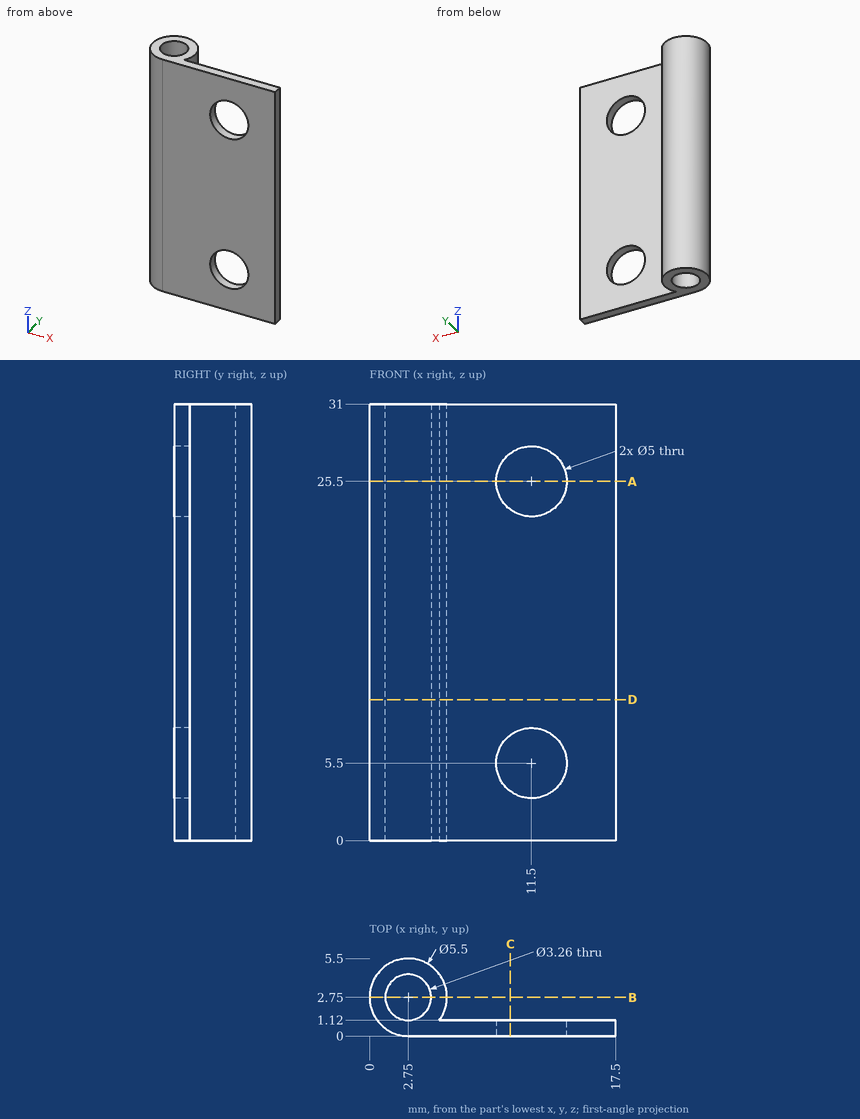
Source: three-view drawing plus pictorial views. Frame: mm from the lowest corner of the part. Round coordinates to 2 decimals unless told otherwise and drop trailing zeros. Order: outer loops, then holes, each group sorted by start corner. A loop starts at its lowest first (then second) coordinate and runs counter-clockwise, first axis right, second up. Notation, with made-up numbers: (27.25, 36) - (84.25, 36) arc R29 ccw to (84.25, 59) - close; hole circle Ø11 at (5, 9). An arc over 180 degrees is marked (long way). Write each question's results on one line, items separated by ' | '.
Item 1: Material intervals for line 1 along Z through (x, y) = (11.5, 0.55); line 2 along Y through (x, z) = (2.75, 7.5), sorted ascending. Write a range as [from, to].
Completed:
line 1: [0, 3], [8, 23], [28, 31] | line 2: [0, 1.12], [4.38, 5.5]
Item 2: First-contact query: pin 1 Ø4 at (x, z) = (14.5, 19.5) entering from +Y; pin 2 Ø4.5 at (x, z) = (11.5, 25.5) entering from +Y. Flat tips, straight axial feed; report the tip coordinate or a pass-through.
Completed:
pin 1: y = 1.12 | pin 2: through
Item 3: Section A-A, the plane z = 25.5. Return the cut outline in (x, y), and give its area (3 significant figures).
Completed:
outline: (2.75, 0) - (9, 0) - (9, 1.12) - (4.96, 1.12) arc R2.75 ccw (long way) to start; (14, 0) - (17.5, 0) - (17.5, 1.12) - (14, 1.12) - close; hole circle Ø3.26 at (2.75, 2.75) | area: 24.6 mm^2
Item 4: Section C-C, the plane x = 10. Return the cut outline in (y, z).
Completed:
outline: (0, 0) - (1.12, 0) - (1.12, 3.5) - (0, 3.5) - close; (0, 7.5) - (1.12, 7.5) - (1.12, 23.5) - (0, 23.5) - close; (0, 27.5) - (1.12, 27.5) - (1.12, 31) - (0, 31) - close
Item 5: Section D-D, the plane z = 10. Return the cut outline in (x, y).
Completed:
outline: (2.75, 0) - (17.5, 0) - (17.5, 1.12) - (4.96, 1.12) arc R2.75 ccw (long way) to start; hole circle Ø3.26 at (2.75, 2.75)
Item 6: Section B-B, the plane y = 2.75. Return the cut outline in (x, z).
Completed:
outline: (0, 0) - (1.12, 0) - (1.12, 31) - (0, 31) - close; (4.38, 0) - (5.5, 0) - (5.5, 31) - (4.38, 31) - close
